Source: CAD feature listing. Evaluate the final solid. Frame: model axes, mm. A direction names the side the tool comes from. Give positions to 0.01 mm unless a question says otherwise; leave off trailing zeros. Order: outer loops, then holes, each group sorted by start corner. A loop starts at its lowest first (then second) coordinate and runs counter-clockwise, first axis right, second up. Notation, with made-up numbers: M 15.5,82 L 74.5,82 A16 cw 74.5,111 Z; hole C 19,34 d7. An arc over 180 degrees is marked long. Return JSON: item names as keys, results as strings.
from build123d import *

# Parameters (mm, degrees)
SKETCH_1_W          = 28
SKETCH_1_H          = 16
EXTRUDE_1_DEPTH     = 4.9
EXTRUDE_2_DEPTH     = 2
SKETCH_3_W          = 6.2
SKETCH_3_H          = 0.8
EXTRUDE_3_DEPTH     = 9
SKETCH_4_R          = 1.1
CUT_EXTRUDE_1_DEPTH = 26.713226169
EXTRUDE_4_DEPTH     = 3.1
CUT_EXTRUDE_2_REACH = 34.408
SKETCH_6_R          = 1.1
EXTRUDE_10_DEPTH    = 2.25
FILLET_1_R          = 3
SKETCH_8_R          = 1.6
CUT_EXTRUDE_3_DEPTH = 31.217464609


with BuildPart() as part:
    # 草图1 → 凸台-拉伸1 (new, symmetric)
    with BuildSketch(Plane.XY):
        Rectangle(SKETCH_1_W, SKETCH_1_H)
    extrude(amount=EXTRUDE_1_DEPTH, both=True)

    # 草图2 → 凸台-拉伸2 (add, symmetric)
    with BuildSketch(Plane.XY):
        with BuildLine():
            Line((8, 8), (11, 8))
            Line((11, 8), (11, 9.5))
            ThreePointArc((11, 9.5), (9.5, 11), (8, 9.5))
            Line((8, 9.5), (8, 8))
        make_face()
    extrude(amount=EXTRUDE_2_DEPTH, both=True)

    # 草图3 → 凸台-拉伸3 (add)
    with BuildSketch(Plane.ZY.offset(14)):
        with Locations((0, 2)):
            Rectangle(SKETCH_3_W, SKETCH_3_H)
        with Locations((0, -3.4)):
            Rectangle(SKETCH_3_W, SKETCH_3_H)
    extrude(amount=EXTRUDE_3_DEPTH)

    # 草图4 → 切除-拉伸1 (cut, through all)
    with BuildSketch(Plane(origin=(0, 2.4, 0), x_dir=(1, 0, 0), z_dir=(0, 1, 0))):
        with Locations(Location((-19, 0, 0), (0, 0, 270))):
            Circle(SKETCH_4_R)
        Polygon((-15.5, 3.1), (-15.5, 2.6), (-22, 2.6), (-23, 1.9), (-23, 3.1), align=None)
        Polygon((-23, -3.1), (-15.5, -3.1), (-15.5, -2.6), (-22, -2.6), (-23, -1.9), align=None)
    extrude(amount=-CUT_EXTRUDE_1_DEPTH, mode=Mode.SUBTRACT)

    # 草图5 → 凸台-拉伸4 (add, symmetric)
    with BuildSketch(Plane.XY):
        with BuildLine():
            Line((-1.5, -8), (-0.7, -8))
            Line((-0.7, -8), (-0.7, -9.8))
            ThreePointArc((-0.7, -9.8), (-1.139339828, -10.860660172), (-2.2, -11.3))
            Line((-2.2, -11.3), (-10.5, -11.3))
            Line((-10.5, -11.3), (-10.5, -10.5))
            Line((-10.5, -10.5), (-2.2, -10.5))
            ThreePointArc((-2.2, -10.5), (-1.705025253, -10.294974747), (-1.5, -9.8))
            Line((-1.5, -9.8), (-1.5, -8))
        make_face()
    extrude(amount=EXTRUDE_4_DEPTH, both=True)

    # 草图6 → 切除-拉伸2 (cut, up to next)
    with BuildSketch(Plane.XZ.offset(11.3), mode=Mode.PRIVATE) as cut_extrude_2_sk1:
        with Locations((-6.5, 0)):
            Circle(SKETCH_6_R)
    cut_extrude_2_tool1 = extrude(cut_extrude_2_sk1.sketch, amount=-CUT_EXTRUDE_2_REACH, mode=Mode.PRIVATE) & part.part
    # 草图6 → 切除-拉伸2 (cut, up to next)
    with BuildSketch(Plane.XZ.offset(11.3), mode=Mode.PRIVATE) as cut_extrude_2_sk2:
        Polygon((-3, 3.1), (-3, 2.6), (-9.5, 2.6), (-10.5, 1.9), (-10.5, 3.1), align=None)
    cut_extrude_2_tool2 = extrude(cut_extrude_2_sk2.sketch, amount=-CUT_EXTRUDE_2_REACH, mode=Mode.PRIVATE) & part.part
    # 草图6 → 切除-拉伸2 (cut, up to next)
    with BuildSketch(Plane.XZ.offset(11.3), mode=Mode.PRIVATE) as cut_extrude_2_sk3:
        Polygon((-10.5, -3.1), (-3, -3.1), (-3, -2.6), (-9.5, -2.6), (-10.5, -1.9), align=None)
    cut_extrude_2_tool3 = extrude(cut_extrude_2_sk3.sketch, amount=-CUT_EXTRUDE_2_REACH, mode=Mode.PRIVATE) & part.part
    add(cut_extrude_2_tool1.solids().sort_by_distance((-6.5, -11.3, 0))[0], mode=Mode.SUBTRACT)
    add(cut_extrude_2_tool2.solids().sort_by_distance((-7.041667, -11.3, 2.80874))[0], mode=Mode.SUBTRACT)
    add(cut_extrude_2_tool3.solids().sort_by_distance((-7.041667, -11.3, -2.80874))[0], mode=Mode.SUBTRACT)

    # 草图7 → 凸台-拉伸10 (add, symmetric)
    with BuildSketch(Plane.XY):
        Polygon((-3, 8), (-2.2, 8), (-2.2, 9.346877402), (24.807562706, 13.408897757), (24.6885785, 14.2), (-3, 10.035552778), align=None)
    extrude(amount=EXTRUDE_10_DEPTH, both=True)

    # 圆角1
    fillet_1_edges = [part.edges().sort_by_distance(p)[0] for p in [
        (14, -8, 0),
        (-14, -8, 0),
        (-14, 8, 0),
        (14, 8, 0),
    ]]
    fillet(fillet_1_edges, radius=FILLET_1_R - 0.0001)  # a hair under: the kernel refuses the full size

    # 草图8 → 切除-拉伸3 (cut, through all)
    with BuildSketch(Plane.XY.offset(4.9)):
        with Locations((-11, 5)):
            Circle(SKETCH_8_R)
        with Locations((11, -5)):
            Circle(SKETCH_8_R)
    extrude(amount=-CUT_EXTRUDE_3_DEPTH, mode=Mode.SUBTRACT)


solid = part.part
1. Ray query, probe 1 along Y at (x, z) = (-11, 1); probe 2 along X at (y, z) = (-3.15, 0); probe 3 along Y at (x, z) = (11.5, -0.25). Return the intervals inside material, ascending.
Evaluation:
{"probe 1": "y = -8 to 3.4, 6.6 to 8", "probe 2": "x = -23 to -20.1, -17.9 to 14", "probe 3": "y = -7.96 to -6.52, -3.48 to 7.96, 11.41 to 12.22"}
2. Section query A-A (x = -16). Return loops of the section in (y, z).
Evaluation:
{"outline": "M -3.8,-2.6 L -3,-2.6 L -3,2.6 L -3.8,2.6 Z; M 1.6,-2.6 L 2.4,-2.6 L 2.4,2.6 L 1.6,2.6 Z"}
3. Section query D-D (y = -8.75). Return loops of the section in (x, z).
Evaluation:
{"outline": "M -1.5,-3.1 L -0.7,-3.1 L -0.7,3.1 L -1.5,3.1 Z"}
4. Section query C-C (y = 5.5). Return loops of the section in (x, z).
Evaluation:
{"outline": "M -13.96,-4.9 L -12.52,-4.9 L -12.52,4.9 L -13.96,4.9 Z; M -9.48,-4.9 L 13.96,-4.9 L 13.96,4.9 L -9.48,4.9 Z"}
5. Draft query along Y for faces 1 (the face through (-17, -3, 0)), 2 (the face through (10.04, 10.9, 0.03)), 3 (the face through (13.1, -7.14, 0.07)), 4 (the face through (11.038, 12.147, 0.031)). Return one class per face: pulls with the +Y half, pulls with the -Y half, needs draft (parallel to the pull), parting line crosses it, or undercut.
Evaluation:
{"face 1": "undercut", "face 2": "undercut", "face 3": "pulls with the -Y half", "face 4": "pulls with the +Y half"}
6. Set-up query: faces 5 (the face through (-17, -3.8, 0)), 6 (the face through (11, 9, 0)), 7 (the face through (-0.7, -9, 0)), 8 (the face through (-3, 9, 0)), 9 (the face through (11.11, 11.35, 0.03)). Return all of +Z, -Z, +X, -X, +Y, -Y with unobstructed straight access to the full face (end or side cutting, diameter ignored); none if empty.
Evaluation:
{"face 5": "+Z, -Z, -X, -Y", "face 6": "+Z, -Z, +X", "face 7": "+Z, -Z, +X, -Y", "face 8": "+Z, -Z, -X, +Y", "face 9": "+Z, -Z"}
7. First-contact query: pin 1 (0.6 mm diameter, centred on x = -15, y = 2, fed in from +Z); pin 2 (3 mm diameter, centred on y = -1, z = -2, fed in from +X); pin 3 (5 mm diameter, centred on x = 10, y = 12, fed in from -Z). Flat tips, straight axial feed; report the tip coordinate or a pass-through.
Evaluation:
{"pin 1": "stops at z = 3.1", "pin 2": "stops at x = 14", "pin 3": "stops at z = -2.25"}
8. Section query B-B (z = -4). Return loops of the section in (x, y).
Evaluation:
{"outline": "M -14,-5 A3 ccw -11,-8 L 11,-8 A3 ccw 14,-5 L 14,5 A3 ccw 11,8 L -11,8 A3 ccw -14,5 Z; hole C -11,5 d3.2; hole C 11,-5 d3.2"}
